Could you check a few things on this drawing? It's one solid part, dimensions in mm from its lowest x, y, z. Round coordinates to 2 decimals unless told otherwise and drop trailing zeros. Loops run counter-clockwise (first coordinate to the right, second up) from the corner with the lowest first, then second, coordinate; pieces in that order, holes last. Notation, with made-up numbers: (88, -31.75) -> (95, -31.75) arc R22 ccw to (95, -14.75) -> close; hole circle Ø9 at (15, -37). An arc over 180 degrees is marked (long way). Put each result on its own line as item: value. Start each with the question number.
1. Imagine slicing it at A-A, the plane y = 115. Please give me the cut outline in (x, z), and give its area (3 significant figures).
2. Imagine slicing it at B-B, the plane x = 237.5. Please give me the cut outline in (y, z).
3. I need wall thicknesses on line 1 (X direction, y = 100.5, z = 1.7); line 2 (Y direction, x = 248, z = 1.5). Which ranges of each line are inside material? Lowest first, please. Write a range as [from, to].
4. I'm going to push a flat-ended pin straight in: P1, Ø0.9, axis at x = 38.5, z = 1, coming from the -Y side. Where does the tip first touch, or does it pass through?
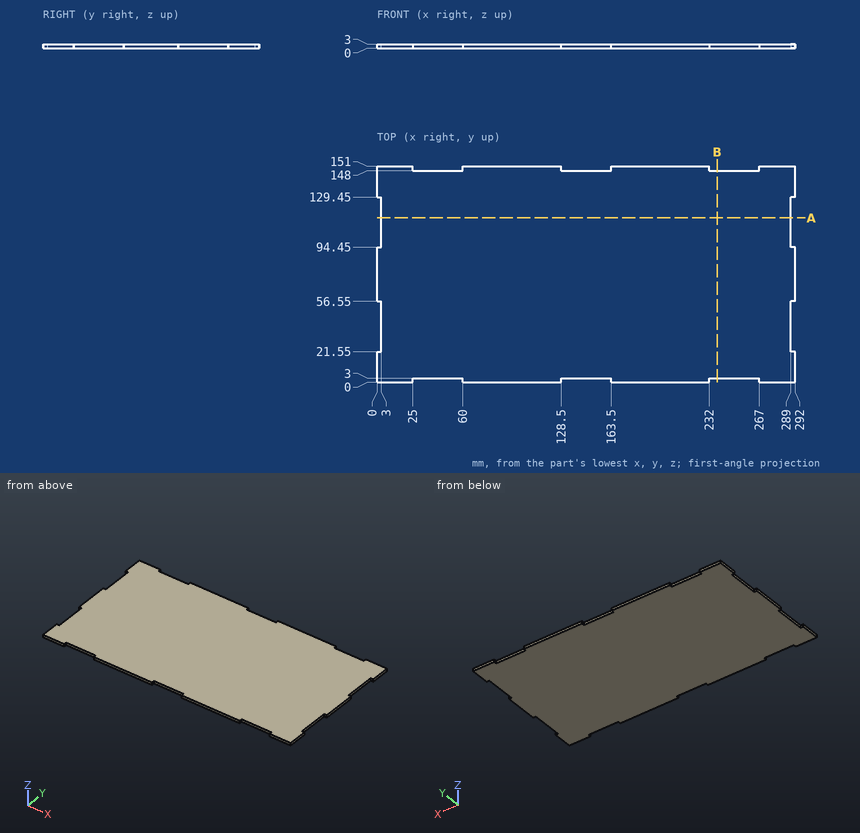
Entries:
1. outline: (3, 0) -> (289, 0) -> (289, 3) -> (3, 3) -> close
1. area: 858 mm^2
2. outline: (3, 0) -> (148, 0) -> (148, 3) -> (3, 3) -> close
3. line 1: [3, 289]
3. line 2: [3, 148]
4. P1: y = 3
